```python
from build123d import *

# Parameters (mm, degrees)
RESSALTO_EXTRUS_O2_DEPTH            = 3
ESCAREADO_PARA_SFHCS_M31_AT_2_COUNT = 2
ESCAREADO_PARA_SFHCS_M31_AT_2_PITCH = 110.642088925
ESCAREADO_PARA_SFHCS_M31_AT_3_COUNT = 2
ESCAREADO_PARA_SFHCS_M31_AT_3_PITCH = 155.41473117
ESCAREADO_PARA_SFHCS_M31_AT_4_COUNT = 2
ESCAREADO_PARA_SFHCS_M31_AT_4_PITCH = 85.967937335
FILETE4_R                           = 5
FILETE6_R                           = 5
FILETE7_R                           = 5
FILETE8_R                           = 5


with BuildPart() as part:
    # Esboço3 → Ressalto-extrusão2 (new body)
    with BuildSketch(Plane(origin=(0, 0, 0), x_dir=(1, 0, 0), z_dir=(0, 1, 0))):
        with BuildLine():
            Line((-21.5, 63.269141943), (-21.5, 37.269141943))
            Line((-21.5, 37.269141943), (-36.5, 37.269141943))
            Line((-36.5, 37.269141943), (-36.5, -2.730858057))
            Line((-36.5, -2.730858057), (-21.5, -2.730858057))
            Line((-21.5, -2.730858057), (-21.5, -12.730858057))
            Line((-21.5, -12.730858057), (21.5, -12.730858057))
            Line((21.5, -12.730858057), (21.5, -2.730858057))
            Line((21.5, -2.730858057), (36.5, -2.730858057))
            Line((36.5, -2.730858057), (36.5, 37.269141943))
            Line((36.5, 37.269141943), (21.5, 37.269141943))
            Line((21.5, 37.269141943), (21.5, 63.269141943))
            ThreePointArc((21.5, 63.269141943), (32.805831499, 66.771318629), (40.152161049, 76.051324532))
            ThreePointArc((40.152161049, 76.051324532), (45.878189612, 72.740578208), (51.332841832, 68.999560502))
            add(Edge.make_bspline(
                [(51.332841832, 68.999560502), (24.845967814, 40.579122115), (79.509348747, 32.775958595)],
                knots=[0, 0, 0, 2.519003886, 2.519003886, 2.519003886], degree=2, weights=[1, 0.306291066, 1]))
            ThreePointArc((79.509348747, 32.775958595), (85.434712449, -9.844283047), (69.971422738, -50))
            add(Edge.make_bspline(
                [(69.971422738, -50), (67.189039214, -47.047402145), (53.286638173, -59)],
                knots=[3.141592654, 3.141592654, 3.141592654, 4.504907102, 4.504907102, 4.504907102], degree=2, weights=[1, 0.776529601, 1]))
            Line((53.286638173, -59), (-53.286638173, -59))
            add(Edge.make_bspline(
                [(-53.286638173, -59), (-67.189039214, -47.047402145), (-69.971422738, -50)],
                knots=[1.778278205, 1.778278205, 1.778278205, 3.141592654, 3.141592654, 3.141592654], degree=2, weights=[1, 0.776529601, 1]))
            ThreePointArc((-69.971422738, -50), (-85.434712449, -9.844283047), (-79.509348747, 32.775958595))
            add(Edge.make_bspline(
                [(-79.509348747, 32.775958595), (-24.845967814, 40.579122115), (-51.332841832, 68.999560502)],
                knots=[0.622588768, 0.622588768, 0.622588768, 3.141592654, 3.141592654, 3.141592654], degree=2, weights=[1, 0.306291066, 1]))
            ThreePointArc((-51.332841832, 68.999560502), (-45.878189612, 72.740578208), (-40.152161049, 76.051324532))
            ThreePointArc((-40.152161049, 76.051324532), (-32.805831499, 66.771318629), (-21.5, 63.269141943))
        make_face()
    extrude(amount=RESSALTO_EXTRUS_O2_DEPTH)

    # Esboço12 → Escareado para SFHCS M31 (revolve, cut)
    with BuildSketch(Plane(origin=(42.983968668, 3, -67.471315665), x_dir=(0, 0, 1), z_dir=(1, 0, 0))):
        Polygon((0, 0), (0, 3), (1.7, 3), (1.7, 1.66), (3.36, 0), align=None)
    escareado_para_sfhcs_m31 = revolve(axis=Axis((42.983968668, 9.35, -67.471315665), (0, -1, 0)), mode=Mode.SUBTRACT)

    # Escareado para SFHCS M31 at 2: Escareado para SFHCS M31 ×2
    with Locations(*[Vector(0.23768589232617374, 0, 0.9713420698132613) * (i * ESCAREADO_PARA_SFHCS_M31_AT_2_PITCH) for i in range(1, ESCAREADO_PARA_SFHCS_M31_AT_2_COUNT)]):
        add(escareado_para_sfhcs_m31, mode=Mode.SUBTRACT)

    # Escareado para SFHCS M31 at 3: Escareado para SFHCS M31 ×2
    with Locations(*[Vector(-0.7223639620597521, 0, 0.6915130557822732) * (i * ESCAREADO_PARA_SFHCS_M31_AT_3_PITCH) for i in range(1, ESCAREADO_PARA_SFHCS_M31_AT_3_COUNT)]):
        add(escareado_para_sfhcs_m31, mode=Mode.SUBTRACT)

    # Escareado para SFHCS M31 at 4: Escareado para SFHCS M31 ×2
    with Locations(*[(-i * ESCAREADO_PARA_SFHCS_M31_AT_4_PITCH, 0, 0) for i in range(1, ESCAREADO_PARA_SFHCS_M31_AT_4_COUNT)]):
        add(escareado_para_sfhcs_m31, mode=Mode.SUBTRACT)

    # Filete4
    filete4_edges = [part.edges().sort_by_distance(p)[0] for p in [
        (21.5, 1.5, -63.269141943),
        (40.152161049, 1.5, -76.051324532),
        (-40.152161049, 1.5, -76.051324532),
        (-21.5, 1.5, -63.269141943),
    ]]
    fillet(filete4_edges, radius=FILETE4_R)

    # Filete6
    filete6_edges = [part.edges().sort_by_distance(p)[0] for p in [
        (69.971422738, 1.5, 50),
        (53.286638173, 1.5, 59),
        (-53.286638173, 1.5, 59),
        (-69.971422738, 1.5, 50),
    ]]
    fillet(filete6_edges, radius=FILETE6_R)

    # Filete7
    filete7_edges = [part.edges().sort_by_distance(p)[0] for p in [
        (-21.5, 1.5, 12.730858057),
        (21.5, 1.5, 12.730858057),
        (21.5, 1.5, 2.730858057),
        (36.5, 1.5, 2.730858057),
        (36.5, 1.5, -37.269141943),
        (21.5, 1.5, -37.269141943),
        (-21.5, 1.5, -37.269141943),
        (-36.5, 1.5, -37.269141943),
        (-36.5, 1.5, 2.730858057),
        (-21.5, 1.5, 2.730858057),
    ]]
    fillet(filete7_edges, radius=FILETE7_R - 0.0001)  # a hair under: the kernel refuses the full size

    # Filete8
    filete8_edges = [part.edges().sort_by_distance(p)[0] for p in [
        (79.509348747, 1.5, -32.775958595),
        (51.332841832, 1.5, -68.999560502),
        (-79.509348747, 1.5, -32.775958595),
        (-51.332841832, 1.5, -68.999560502),
    ]]
    fillet(filete8_edges, radius=FILETE8_R)


solid = part.part
```
For this review, take the finished solid that the model builds, in its own axes (mm). A direction names the side the tool comes from. Round coordinates to 2 decimals unless told otherwise and drop trailing zeros. Write each loop counter-clockwise with the first axis right and the second up, starting at its lowest first coordinate (ties: lowest second). Pieces come first, ordered by that corner, then holes. Notation, with made-up numbers: (-2, -17.75) - (16, -17.75) arc R21 ccw to (16, -2.75) - close; hole circle Ø7 at (-5, -5.75). An arc over 180 degrees is marked (long way). Put each result on its own line as item: value.
Q1. We need section A-A (z = -23). Give the boundary of the cut face in (x, y), and give its area (3 significant figures).
Solved:
outline: (-82.87, 0) - (-36.5, 0) - (-36.5, 3) - (-82.87, 3) - close; (36.5, 0) - (82.87, 0) - (82.87, 3) - (36.5, 3) - close
area: 278 mm2
Q2. Mouldability with a two-part tool opening along X and no side actions: class faces 4 (the face through (85.516, 1.479, 9.111)), 5 (the face through (20, 1.5, 11.3)), 6 (the face through (1, 3, 21)), 7 (the face through (-85.39, 1.48, 10.24)) as released by +X, released by -X, zero draft, split by the parting line, or undercut.
Solved:
face 4: released by +X
face 5: undercut
face 6: zero draft
face 7: released by -X
Q3. Machinability: for faces 1 (the face through (1, 0, 21)), 2 (the face through (-32.7, 1.5, -66.7)), 3 (the face through (-23, 1.52, 4.16)), which of the approach directions +Z, -Z, +X, -X, +Y, -Y give a long, thin tool a straight path to every point of the face, cutting with its end or side? Answer none if there is none.
Solved:
face 1: +Z, -Z, +X, -X, -Y
face 2: -Z, +Y, -Y
face 3: +Y, -Y
Q4. Wall thickness on probe 1 along X at (y, z) = (0.65, 40); probe 2 along X at (y, z) = (2.3, 41); probe 3 along Z at (x, y) = (-77, 0.65): over which ranges is each line inside the solid? List them lowest first.
Solved:
probe 1: x = -76.13 to -70.98, -67.58 to 67.58, 70.98 to 76.13
probe 2: x = -75.6 to -71.75, -66.82 to 66.82, 71.75 to 75.6
probe 3: z = -33.3 to 38.3
Q5. Insertion check: pin 1 Ø2 at (x, z) = (-42.98, -67.47) entering from -Y; pin 2 Ø0.9 at (y, z) = (2, -53) entering from -X; pin 3 Ø0.9 at (y, z) = (1.5, -22) entering from +X; pin 4 Ø0.9 at (y, z) = (1, -47) entering from +X. Each pin has a flat end and moves straight along its axis. Give the tip position at first contact, or say it passes through.
Solved:
pin 1: passes through
pin 2: stops at x = -53.1
pin 3: stops at x = 83.26
pin 4: stops at x = 57.49
Q6. We need section D-D (x = -10). Give the boundary of the cut face in (y, z), and give its area (3 significant figures).
Solved:
outline: (0, 12.73) - (3, 12.73) - (3, 59) - (0, 59) - close
area: 139 mm2
Q7. We need section C-C (z = -6.5). Give the boundary of the cut face in (x, y).
Solved:
outline: (-85.75, 0) - (-36.5, 0) - (-36.5, 3) - (-85.75, 3) - close; (36.5, 0) - (85.75, 0) - (85.75, 3) - (36.5, 3) - close
Q8. We need section B-B (y = 2.15). Count the separate pieces of the cut face and the enclosed holes in it, and give its area (3 significant figures).
Solved:
separate pieces: 1
enclosed holes: 4
area: 14,000 mm2
